Part model, mm, in its own coordinate system. A direction names the side the tool comes from. Coordinates: 2 decimals unless noted, no trailing zeros. Order: outer loops, then holes, each group sorted by start corner. A loop starts at its lowest first (then second) coordinate and runs counter-clockwise, first axis right, second up.
from build123d import *

# Parameters (mm, degrees)
SKETCH1_R                                       = 2.6
SKETCH1_R_2                                     = 6.25
SKETCH1_W                                       = 4.9
SKETCH1_H                                       = 45
BOSS_EXTRUDE1_DEPTH                             = 13.5
SKETCH1_3_R                                     = 6.25
BOSS_EXTRUDE2_DEPTH                             = 0.6
BOSS_EXTRUDE3_START                             = -13.5
SKETCH1_4_W                                     = 4.9
SKETCH1_4_H                                     = 45
BOSS_EXTRUDE3_DEPTH                             = 1
CSK_FOR_M5_FLAT_HEAD_MACHINE_SCREW2_D           = 5.3
CSK_FOR_M5_FLAT_HEAD_MACHINE_SCREW2_CSINK_D     = 10.4
CSK_FOR_M5_FLAT_HEAD_MACHINE_SCREW2_CSINK_ANGLE = 90
CUT_EXTRUDE1_DEPTH                              = 46.263119645


with BuildPart() as part:
    # Sketch1 → Boss-Extrude1 (new body)
    # profile 1 of 3: a face of its own
    with BuildSketch(Plane(origin=(0, 0, 0), x_dir=(1, 0, 0), z_dir=(0, 1, 0))):
        with BuildLine():
            Line((-2.45, 22.5), (-12.5, 22.5))
            ThreePointArc((-12.5, 22.5), (-17.644957554, 21.074929257), (-21.323529412, 17.205882353))
            Line((-21.323529412, 17.205882353), (-35.911764706, -10.147058824))
            ThreePointArc((-35.911764706, -10.147058824), (-36.091023102, -14.480531969), (-32.815789474, -17.323763889))
            Line((-32.815789474, -17.323763889), (-15.131578947, -22.147527779))
            ThreePointArc((-15.131578947, -22.147527779), (-13.827539493, -22.411490246), (-12.5, -22.5))
            Line((-12.5, -22.5), (-2.45, -22.5))
            Line((-2.45, -22.5), (-2.45, 22.5))
        make_face()
        with Locations(Location((-31.5, -12.5, 0), (0, 0, 270))):
            Circle(SKETCH1_R, mode=Mode.SUBTRACT)
        with Locations(Location((-12.5, -12.5, 0), (0, 0, 270))):
            Circle(SKETCH1_R_2, mode=Mode.SUBTRACT)
        with Locations(Location((-12.5, 12.5, 0), (0, 0, 270))):
            Circle(SKETCH1_R_2, mode=Mode.SUBTRACT)
    # profile 2 of 3: a face of its own
    with BuildSketch(Plane(origin=(0, 0, 0), x_dir=(1, 0, 0), z_dir=(0, 1, 0))):
        Rectangle(SKETCH1_W, SKETCH1_H)
    # profile 3 of 3: a face of its own
    with BuildSketch(Plane(origin=(0, 0, 0), x_dir=(1, 0, 0), z_dir=(0, 1, 0))):
        with BuildLine():
            Line((12.5, 22.5), (2.45, 22.5))
            Line((2.45, 22.5), (2.45, -22.5))
            Line((2.45, -22.5), (12.5, -22.5))
            ThreePointArc((12.5, -22.5), (17.644957554, -21.074929257), (21.323529412, -17.205882353))
            Line((21.323529412, -17.205882353), (35.911764706, 10.147058824))
            ThreePointArc((35.911764706, 10.147058824), (36.091023102, 14.480531969), (32.815789474, 17.323763889))
            Line((32.815789474, 17.323763889), (15.131578947, 22.147527779))
            ThreePointArc((15.131578947, 22.147527779), (13.827539493, 22.411490246), (12.5, 22.5))
        make_face()
        with Locations(Location((12.5, -12.5, 0), (0, 0, 270))):
            Circle(SKETCH1_R_2, mode=Mode.SUBTRACT)
        with Locations(Location((12.5, 12.5, 0), (0, 0, 270))):
            Circle(SKETCH1_R_2, mode=Mode.SUBTRACT)
        with Locations(Location((31.5, 12.5, 0), (0, 0, 270))):
            Circle(SKETCH1_R, mode=Mode.SUBTRACT)
    extrude(amount=-BOSS_EXTRUDE1_DEPTH)

    # Sketch1<3> → Boss-Extrude2 (add)
    with BuildSketch(Plane(origin=(0, 0, 0), x_dir=(1, 0, 0), z_dir=(0, 1, 0))):
        with Locations(Location((-12.5, 12.5, 0), (0, 0, 270))):
            Circle(SKETCH1_3_R)
        with Locations(Location((12.5, 12.5, 0), (0, 0, 270))):
            Circle(SKETCH1_3_R)
        with Locations(Location((12.5, -12.5, 0), (0, 0, 270))):
            Circle(SKETCH1_3_R)
        with Locations(Location((-12.5, -12.5, 0), (0, 0, 270))):
            Circle(SKETCH1_3_R)
    extrude(amount=-BOSS_EXTRUDE2_DEPTH)

    # Sketch1<4> → Boss-Extrude3 (add)
    with BuildSketch(Plane(origin=(0, 0, 0), x_dir=(1, 0, 0), z_dir=(0, 1, 0)).offset(BOSS_EXTRUDE3_START)):
        Rectangle(SKETCH1_4_W, SKETCH1_4_H)
    extrude(amount=-BOSS_EXTRUDE3_DEPTH)

    # CSK for M5 Flat Head Machine Screw2 (through all)
    with Locations(Plane(origin=(0, 0, 0), x_dir=(1, 0, 0), z_dir=(0, 1, 0))):
        with Locations((0, 16), (0, 0), (0, -16)):
            CounterSinkHole(CSK_FOR_M5_FLAT_HEAD_MACHINE_SCREW2_D / 2, CSK_FOR_M5_FLAT_HEAD_MACHINE_SCREW2_CSINK_D / 2, counter_sink_angle=CSK_FOR_M5_FLAT_HEAD_MACHINE_SCREW2_CSINK_ANGLE)

    # Sketch8 → Cut-Extrude1 (cut, symmetric)
    with BuildSketch(Plane.XY):
        with BuildLine():
            ThreePointArc((32.794095226, -7.568721494), (35.466766701, -5.782899508), (36.5, -2.739092363))
            Line((36.5, -2.739092363), (36.5, -13.5))
            Line((36.5, -13.5), (10, -13.5))
            ThreePointArc((10, -13.5), (10.652630961, -13.457224307), (11.294095226, -13.329629131))
            Line((11.294095226, -13.329629131), (32.794095226, -7.568721494))
        make_face()
    cut_extrude1 = extrude(amount=CUT_EXTRUDE1_DEPTH, both=True, mode=Mode.SUBTRACT)

    # Mirror1: Cut-Extrude1 across plane
    add(cut_extrude1.mirror(Plane(origin=(0, 0, 0), x_dir=(0, 0, 1), z_dir=(1, 0, 0))), mode=Mode.SUBTRACT)


solid = part.part
Q1. Wall check: line 1 along Z through (x, y) = (-12.5, -10.5); line 2 along X through (y, z) = (-4.75, 14); line 3 along X through (y, z) = (-5.75, -12.5). Give the ranges that are in metal, low to high.
Results list:
line 1: z = -22.5 to -18.75, -6.25 to 6.25, 18.75 to 22.5
line 2: x = -36.08 to -33.62, -29.38 to -18.57, -6.43 to -1.74, 1.74 to 6.43, 18.57 to 23.03
line 3: x = -23.83 to -18.75, -6.25 to 6.25, 18.75 to 28.9, 34.1 to 35.49
Q2. Cut at B-B on x = -31.5. Write the cut outline in (y, z) (3 decimals), and give its area (3 significant figures).
Results list:
outline: (-7.915, 1.875) - (0, 1.875) - (0, 9.9) - (-7.915, 9.9) - close; (-7.915, 15.1) - (0, 15.1) - (0, 17.683) - (-7.915, 17.683) - close
area: 84.0 mm2
Q3. Mould opens along X. For faces 4 (the face through (0.601, -2.426, -13.292)), 5 (the face through (-13.85, -6.41, 22.41)), 6 (the face through (17.6, -6.4, 21.1)), 7 (the face through (-6.3, -7, 11.7)) say: pulls with the +X half, pulls with the -X half, needs draft (parallel to the pull), parting line crosses it, or undercut.
Results list:
face 4: undercut
face 5: pulls with the -X half
face 6: pulls with the +X half
face 7: undercut
Q4. Cut at A-A on z = -16. Write the cut outline in (x, y), and give its area (3 significant figures).
Results list:
outline: (-21.97, -10.47) - (-17.68, -11.62) - (-17.68, -0.6) - (-7.32, -0.6) - (-7.32, -13.5) - (-2.65, -13.5) - (-2.65, -2.55) - (-5.2, 0) - (-21.97, 0) - close; (2.65, -13.5) - (7.32, -13.5) - (7.32, -0.6) - (17.68, -0.6) - (17.68, -11.62) - (32.79, -7.57) arc R5 ccw to (35.07, -6.24) - (35.07, 0) - (5.2, 0) - (2.65, -2.55) - close
area: 340 mm2
Q5. Pin check, flat tips, straight feed: pin 1 Ø7 at (x, z) = (0, 0) entering from +Y; pin 2 Ø8 at (x, y) = (-25.5, -10) entering from -Z (3 decimals); pin 3 Ø11 at (x, z) = (12.5, 12.5) entering from -Y; pin 4 Ø4 at (x, z) = (0, 16) entering from +Y. Stop position of each tip, or through.
Results list:
pin 1: stops at y = -1.7
pin 2: stops at z = -16.875
pin 3: stops at y = -0.6
pin 4: passes through
Q6. Cut at C-C on z = 0. Write the cut outline in (x, y).
Results list:
outline: (-30.5, -8.18) - (-11.29, -13.33) arc R5 ccw to (-10, -13.5) - (-2.65, -13.5) - (-2.65, -2.55) - (-5.2, 0) - (-30.5, 0) - close; (2.65, -13.5) - (10, -13.5) arc R5 ccw to (11.29, -13.33) - (30.5, -8.18) - (30.5, 0) - (5.2, 0) - (2.65, -2.55) - close
Q7. Which spindle directions (+Z, -Z, +X, -X, +Y, -Y) get a long thin tool onto all of the face, cutting with end or side? Do faces 1 (the face through (5, -13.5, 0)), 2 (the face through (-34.95, -6.36, 12.35)), 3 (the face through (-6.3, -7, -13.3)). Say none if no direction does.
Results list:
face 1: +Z, -Z, +X, -Y
face 2: +Z, -Z, -X, -Y
face 3: -Y
